Study the drawing (mm; zero at the part's minimum x, y, z) and answer. A direction names the side the tool comes from. Give positions to 0.01 mm unless a question says otherwise; leave off trailing zeros. Loops run counter-clockwise (first coordinate to the right, second up) from the corner with the lowest first, then second, coordinate; pieces in that order, holes last. Notation, with made-up numbers: (67, -8) - (106, -8) arc R24 ccw to (106, 19) - close; hole circle Ø1 at (40.25, 77.5). An arc over 180 degrees is marked (long way). Answer in a Markdown table with one row per item. Add a question column.
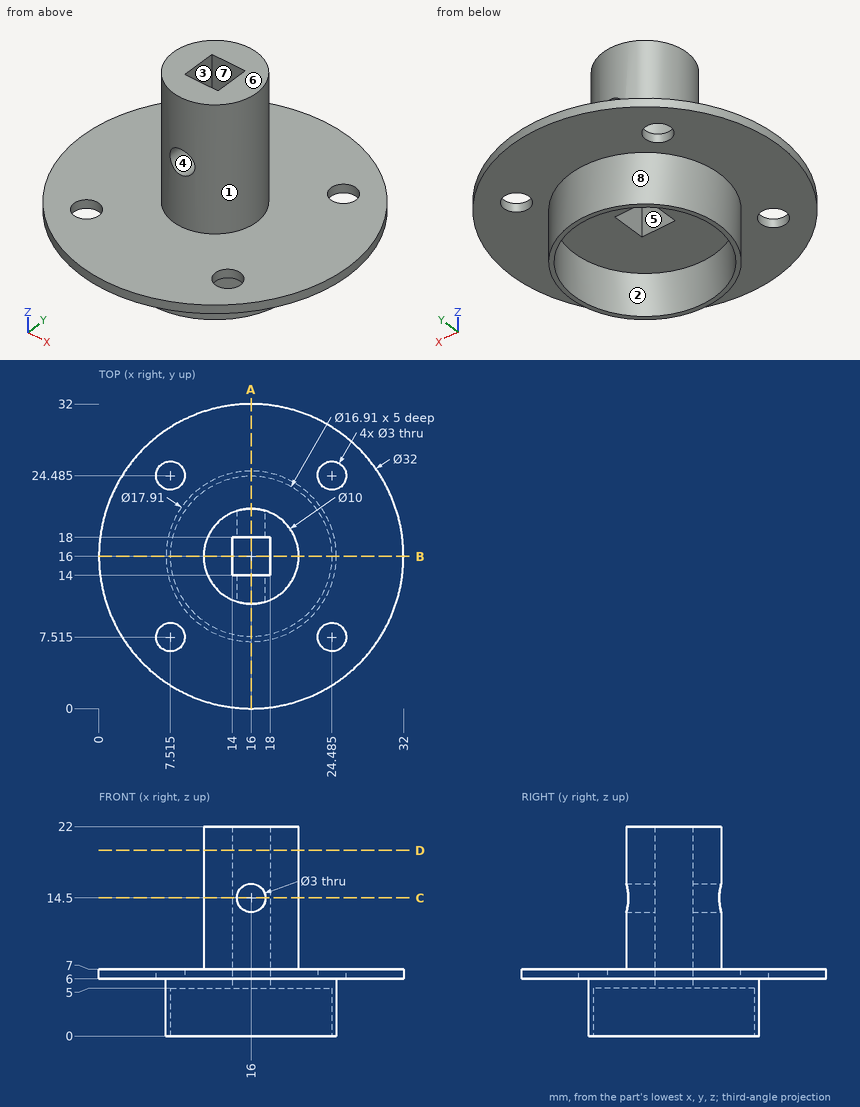
(1) A cutting plane is placed at D-D on z = 19.5. Determine the outline of the cut face in (x, y).
(2) The mould has two halves that part along X. Classify the marked faces 5, 6, 7 and 8: pulls with the +X half, pulls with the -X half, needs draft (parallel to the pull), parting line crosses it, or undercut.
(3) A cutting plane is placed at B-B on y = 16. Determine the outline of the cut face in (x, z) (1 decimal), plus the area to 3 significant figures.
(4) A cutting plane is placed at C-C on z = 14.5. Determine the outline of the cut face in (x, y).
(5) A cutting plane is placed at A-A on x = 16. Determine the outline of the cut face in (y, z) (1 decimal).
(6) Given pin 1 Ø5 at (x, y) = (26, 13) entering from +Z; pin 2 Ø1.2 at (x, z) = (16.5, 12.5) entering from -Y; pin 3 Ø3 at (y, z) = (16.5, 15.5) entering from -X; pin 4 Ø2.5 at (x, y) = (7.51, 24.49) entering from +Z, each flat-ended and moving along its own axis, determine where each tip first touches the part or whether it passes through.
(7) Find the intervals of material crossed by line 1 along Z through (x, y) = (16, 18.7); line 2 along Z through (x, y) = (30.5, 14.5); line 3 along Y through (x, z) = (17, 17.5), in increasing order. Write a range as [from, to].
(8) A tool of negligible diameter and unlimited length cuts with its end or side. For the marked faces 1, 2, 3 and 4, from which of +Z, -Z, +X, -X, +Y, -Y can it reach the whole face along a straight path? Write none if from no direction.
Evaluation:
| question | item | result |
|---|---|---|
| 1 | outline | circle Ø10 at (16, 16); hole (14, 14) - (18, 14) - (18, 18) - (14, 18) - close |
| 2 | face 5 | undercut |
| 2 | face 6 | needs draft |
| 2 | face 7 | undercut |
| 2 | face 8 | parting line crosses it |
| 3 | outline | (0, 6) - (7, 6) - (7, 0) - (7.5, 0) - (7.5, 5) - (14, 5) - (14, 22) - (11, 22) - (11, 7) - (0, 7) - close; (18, 5) - (24.5, 5) - (24.5, 0) - (25, 0) - (25, 6) - (32, 6) - (32, 7) - (21, 7) - (21, 22) - (18, 22) - close |
| 3 | area | 137 mm² |
| 4 | outline | (14, 14) - (14, 18) - (14.5, 18) - (14.5, 20.77) arc R5 ccw to (14.5, 11.23) - (14.5, 14) - close; (17.5, 11.23) arc R5 ccw to (17.5, 20.77) - (17.5, 18) - (18, 18) - (18, 14) - (17.5, 14) - close |
| 5 | outline | (0, 6) - (7, 6) - (7, 0) - (7.5, 0) - (7.5, 5) - (14, 5) - (14, 13) - (11, 13) - (11, 7) - (0, 7) - close; (11, 16) - (14, 16) - (14, 22) - (11, 22) - close; (18, 5) - (24.5, 5) - (24.5, 0) - (25, 0) - (25, 6) - (32, 6) - (32, 7) - (21, 7) - (21, 13) - (18, 13) - close; (18, 16) - (21, 16) - (21, 22) - (18, 22) - close |
| 6 | pin 1 | stops at z = 7 |
| 6 | pin 2 | stops at y = 11 |
| 6 | pin 3 | stops at x = 11 |
| 6 | pin 4 | passes through |
| 7 | line 1 | z = [5, 13], [16, 22] |
| 7 | line 2 | z = [6, 7] |
| 7 | line 3 | y = [11.1, 14], [18, 20.9] |
| 8 | face 1 | +Z |
| 8 | face 2 | -Z |
| 8 | face 3 | +Z, -Z |
| 8 | face 4 | +Y, -Y |
